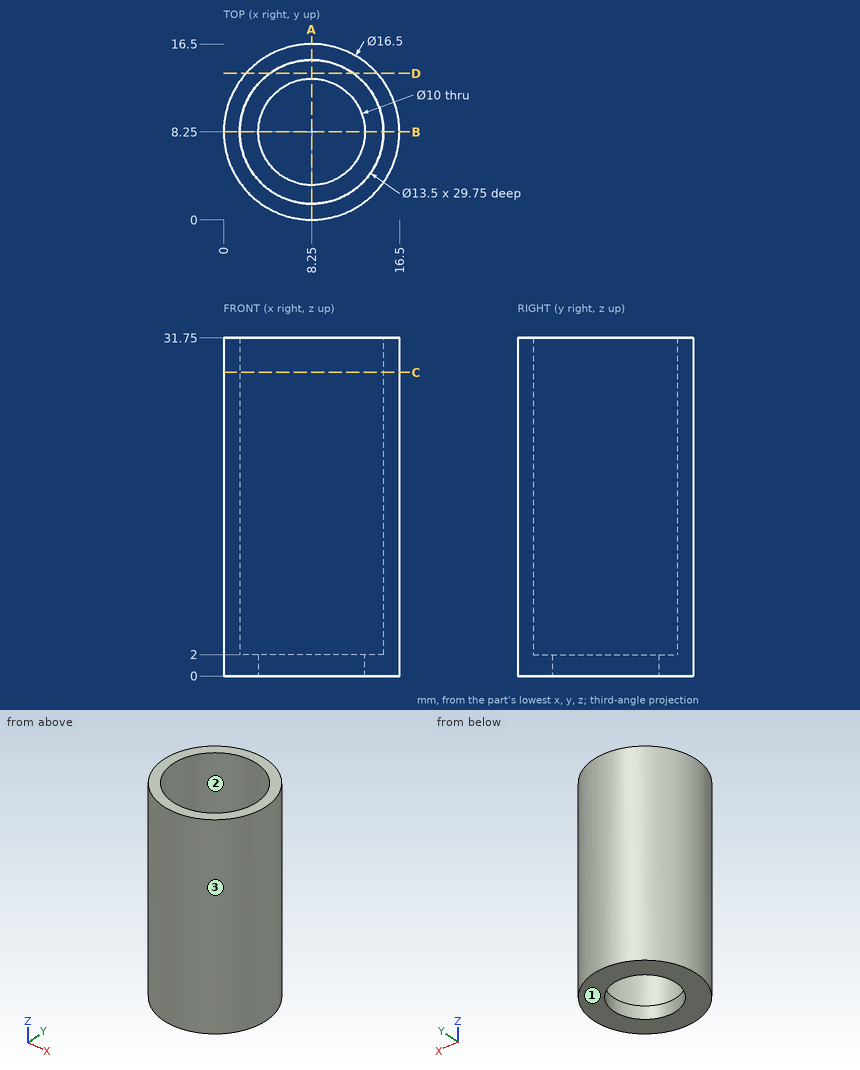
Verification items for this drawing (mm, ordinates from the low corner). Round coordinates to 2 decimals unless told otherwise and drop trailing zeros. Order: outer loops, then holes, each group sorted by start corner. A loop starts at its lowest first (then second) coordinate and runs counter-clockwise, first axis right, second up. Notation, with made-up numbers: (37, 76.5) - (76, 76.5) arc R4 cw to (76, 81.5) - close; hole circle Ø4 at (-13, 17.5). An arc over 180 degrees is marked (long way). Use CSV: the item, a comma, the result in double quotes.
(1) Mould release check, pull along X, two halves, no side actions. Record for the marked faces 1, 2 and 3: released by +X, released by -X, zero draft, split by the parting line, or undercut.
Entries:
face 1,"zero draft"
face 2,"undercut"
face 3,"split by the parting line"
(2) Section check C-C on z = 28.5. Record the boundary of the cut face in (x, y).
Entries:
outline,"circle Ø16.5 at (8.25, 8.25); hole circle Ø13.5 at (8.25, 8.25)"
(3) Thickness scan on probe 1 along Y at (x, z) = (8.25, 0.8); probe 2 along Y at (x, z) = (9.75, 19.5); probe 3 along X at (y, z) = (6.5, 2.5). Record the ranges inside material, lowest first. Write a range as from..to.
Entries:
probe 1,"0..3.25, 13.25..16.5"
probe 2,"0.14..1.67, 14.83..16.36"
probe 3,"0.19..1.73, 14.77..16.31"
(4) Section check A-A on x = 8.25. Record the boundary of the cut face in (y, z), and give its area (3 significant figures).
Entries:
outline,"(0, 0) - (3.25, 0) - (3.25, 2) - (1.5, 2) - (1.5, 31.75) - (0, 31.75) - close; (13.25, 0) - (16.5, 0) - (16.5, 31.75) - (15, 31.75) - (15, 2) - (13.25, 2) - close"
area,"102 mm^2"
(5) Gauge pin test, flat ends, axial feed: pin 1 Ø3 at (y, z) = (13.5, 6) entering from -X; pin 2 Ø1.5 at (x, z) = (14.5, 27) entering from -Y; pin 3 Ø1 at (y, z) = (4.5, 25) entering from +X. Record the tip position at first contact, or that the pin passes through.
Entries:
pin 1,"x = 0.9"
pin 2,"y = 2.1"
pin 3,"x = 15.83"
(6) Section check D-D on y = 13.75. Record the boundary of the cut face in (x, z).
Entries:
outline,"(2.1, 0) - (14.4, 0) - (14.4, 31.75) - (12.16, 31.75) - (12.16, 2) - (4.34, 2) - (4.34, 31.75) - (2.1, 31.75) - close"
